Answer from the drawing. Dimensions are ordinates in mm from the lowest x, y and z of the part. Give positions to 0.01 mm unless a question says otherwise; leave off trailing zeros. Order: outer loops, then holes, each group sorted by start corner. A loop starts at its lowest first (then second) coordinate and runs counter-clockwise, first axis right, second up.
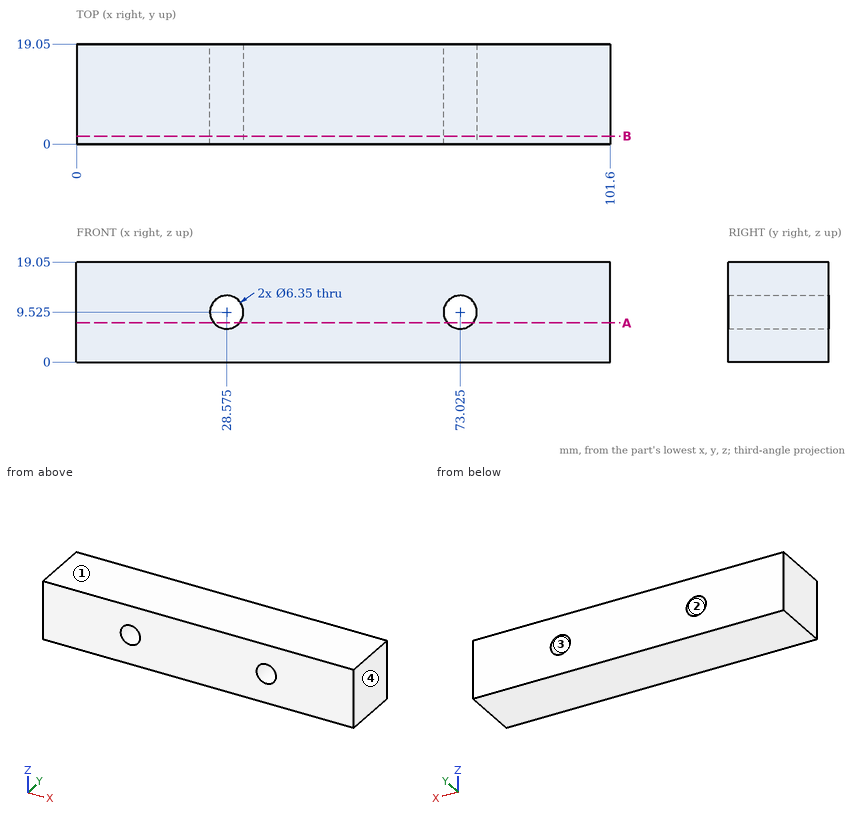
1) Consider L1, parallel to X at y = 7.25, z = 8.25; L2, parallel to X at y = 3.5, z = 11.75; L3, parallel to Z at x = 73, y = 2.5. Determine where each line is inside the solid, lowest interval first.
Final values:
L1: x = 0 to 25.67, 31.48 to 70.12, 75.93 to 101.6
L2: x = 0 to 26.31, 30.84 to 70.76, 75.29 to 101.6
L3: z = 0 to 6.35, 12.7 to 19.05
2) The part is cut by section B-B on y = 1.5. Determine the outline of the cut face in (x, z) (3 decimals), and give its area (3 significant figures).
Final values:
outline: (0, 0) - (101.6, 0) - (101.6, 19.05) - (0, 19.05) - close; hole circle Ø6.35 at (28.575, 9.525); hole circle Ø6.35 at (73.025, 9.525)
area: 1,870 mm2
3) For a pull along X with two mould halves and no side action, classify the marked faces 1, 2, 3 and 4 as released by +X, released by -X, zero draft, split by the parting line, or undercut.
Final values:
face 1: zero draft
face 2: undercut
face 3: undercut
face 4: released by +X
4) The part is cut by section A-A on z = 7.5. Determine the outline of the cut face in (x, y).
Final values:
outline: (0, 0) - (26.13, 0) - (26.13, 19.05) - (0, 19.05) - close; (31.02, 0) - (70.58, 0) - (70.58, 19.05) - (31.02, 19.05) - close; (75.47, 0) - (101.6, 0) - (101.6, 19.05) - (75.47, 19.05) - close
